Verification items for the finished model (mm, model axes). Coordinates: 2 decimals unless noted, no trailing zeros. Order: outer loops, then holes, each group sorted by start corner. A loop starts at its lowest first (then second) coordinate and runs counter-clockwise, first axis right, second up. Notation, with made-up numbers: (60, 14.5) -> (79, 14.5) arc R24 ccw to (79, 48.5) -> close; hole circle Ø1 at (72.5, -31). An arc over 180 degrees is marked (long way). Write item = value, one per line. Start each with the question number.
from build123d import *

# Parameters (mm, degrees)
SKETCH2_R               = 2
SKETCH2_W               = 20.1
SKETCH2_H               = 40.1
BOSS_EXTRUDE1_DEPTH     = 3.175
CUT_EXTRUDE1_DEPTH      = 122.340185532
CUT_EXTRUDE1_DEPTH_BACK = 122.340185532
SKETCH3_R               = 1.6


with BuildPart() as part:
    # Sketch2 → Boss-Extrude1 (new body)
    with BuildSketch(Plane(origin=(0, 0, 0), x_dir=(1, 0, 0), z_dir=(0, 1, 0))):
        with BuildLine():
            Line((-13, 0), (-13, -61.6))
            Line((-13, -61.6), (-4, -116.6))
            ThreePointArc((-4, -116.6), (0, -120.6), (4, -116.6))
            Line((4, -116.6), (13, -61.6))
            Line((13, -61.6), (13, 0))
            ThreePointArc((13, 0), (0, 13), (-13, 0))
        make_face()
        with Locations(Location((-5, 4.5, 0), (0, 0, 270))):
            Circle(SKETCH2_R, mode=Mode.SUBTRACT)
        with Locations(Location((-5, -45.6, 0), (0, 0, 270))):
            Circle(SKETCH2_R, mode=Mode.SUBTRACT)
        with Locations(Location((5, -45.6, 0), (0, 0, 90))):
            Circle(SKETCH2_R, mode=Mode.SUBTRACT)
        with Locations(Location((5, 4.5, 0), (0, 0, 90))):
            Circle(SKETCH2_R, mode=Mode.SUBTRACT)
        with Locations((0, -20.55)):
            Rectangle(SKETCH2_W, SKETCH2_H, mode=Mode.SUBTRACT)
    extrude(amount=BOSS_EXTRUDE1_DEPTH)

    # Sketch3 → Cut-Extrude1 (cut, two sides: drawn at the far end of the back side and taken through both)
    with BuildSketch(Plane(origin=(0, 3.175, 0), x_dir=(1, 0, 0), z_dir=(0, 1, 0)).offset(-CUT_EXTRUDE1_DEPTH_BACK)):
        with Locations(Location((10, -58.9, 0), (0, 0, 270))):
            Circle(SKETCH3_R)
        with Locations(Location((10, -51.4, 0), (0, 0, 270))):
            Circle(SKETCH3_R)
        with Locations(Location((-10, -58.9, 0), (0, 0, 270))):
            Circle(SKETCH3_R)
        with Locations(Location((-10, -51.4, 0), (0, 0, 270))):
            Circle(SKETCH3_R)
    extrude(amount=CUT_EXTRUDE1_DEPTH + CUT_EXTRUDE1_DEPTH_BACK, mode=Mode.SUBTRACT)


solid = part.part
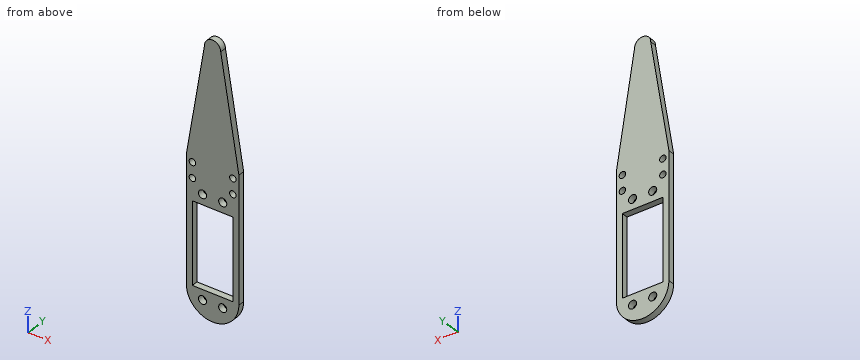
Item 1: Section check D-D (z = 108). Record the boundary of the cut face in (x, y) (3 decimals).
Item 2: Section check C-C (z = -5). Record the boundary of the cut face in (x, y) (1 decimal), then the cut area to 3 significant figures.
Item 3: Thickness scan on line 1 (X direction, y = 2.4, z = 58.9); line 2 (X direction, y = 2.2, z = 45.6); line 3 (X direction, y = 1, z = 40). Record the ranges inside material, lowest first.
Item 4: Gauge pin test, flat ends, axial feed: P1, Ø1.5, axis at x = 4.5, y = 1, coming from the -Z side; P2, Ø3, axis at x = -10, z = 58.9, coming from the +Y side. Record the tip position at first contact, or that the pin passes through.
Item 5: Section check A-A (z = 45.6). Record the boundary of the cut face in (x, y) (3 decimals), then the cut area to 4 significant figures.
Item 6: Section check B-B (y = 1.3). State how many separate pieces and enclosed holes the cut face has, then the cut area to 3 significant figures.
Filled sheet:
q1.outline = (-5.407, 0) -> (5.407, 0) -> (5.407, 3.175) -> (-5.407, 3.175) -> close
q2.outline = (-12, 0) -> (-6.9, 0) -> (-6.9, 3.2) -> (-12, 3.2) -> close; (-3.1, 0) -> (3.1, 0) -> (3.1, 3.2) -> (-3.1, 3.2) -> close; (6.9, 0) -> (12, 0) -> (12, 3.2) -> (6.9, 3.2) -> close
q2.area = 51.6 mm^2
q3.line_1 = -13 to -11.6, -8.4 to 8.4, 11.6 to 13
q3.line_2 = -13 to -7, -3 to 3, 7 to 13
q3.line_3 = -13 to -10.05, 10.05 to 13
q4.P1 = -12.45
q4.P2 = through
q5.outline = (-13, 0) -> (-7, 0) -> (-7, 3.175) -> (-13, 3.175) -> close; (-3, 0) -> (3, 0) -> (3, 3.175) -> (-3, 3.175) -> close; (7, 0) -> (13, 0) -> (13, 3.175) -> (7, 3.175) -> close
q5.area = 57.15 mm^2
q6.separate_pieces = 1
q6.enclosed_holes = 9
q6.area = 1,940 mm^2
